Autodesk Inventor part; units mm, degrees
ref_plane "Flange Pattern Plane" through (19.05, 7.9375, -4.5466) normal (0, 1, 0) x (1, 0, 0)
ref_plane "YZ Plane" through (0, 0, 0) normal (1, 0, 0) x (0, 1, 0)
ref_plane "XZ Plane" through (0, 0, 0) normal (0, 1, 0) x (-1, 0, 0)
sketch "Sketch1" plane through (0, 0, 0) normal (0, 1, 0) x (-1, 0, 0)
  line L0 (-19.05, 0) -> (19.05, 0)
  line L1 (19.05, 0) -> (19.05, -25.4)
  line L2 (19.05, -25.4) -> (-19.05, -25.4)
  line L3 (-19.05, -25.4) -> (-19.05, 0)
  line L4 (19.05, 0) -> (-19.05, -25.4) construction
  point P0 (0, 0)
  point P1 (0, 0)
  dimension "d0" = 38.1
  dimension "d1" = 25.4
extrude "Plate1" add sketch "Sketch1" along normal blind 1.5875
sketch "Sketch2" plane through (17.4625, 0, -25.4) normal (1, 0, 0) x (0, 1, 0)
  line L0 (0, 25.4) -> (0, 0)
  line L1 (0, 0) -> (14.2875, 0)
  line L2 (14.2875, 0) -> (14.2875, 25.4)
  line L3 (14.2875, 25.4) -> (0, 25.4)
edge flange "Flanges" height 12.7 angle 90 thickness 1.5875 bend radius 0.7937 thickness toward (1, 0, 0) relief tear relief width 1.5875 relief depth 0.7937 corner gap 1.5875 corner form 0 edges at (19.05, 1.5875, -12.7) (-19.05, 1.5875, -12.7) wall of the first edge with corners at (17.4625, 0, 0) (17.4625, 0, -25.4) (17.4625, 14.2875, -25.4) (17.4625, 14.2875, 0)
bend "Bend1"
corner "Corner1"
sketch "Sketch3" plane through (19.05, 2.3813, -25.4) normal (1, 0, 0) x (0, 0, -1)
  line L0 (-20.8534, 7.8677) -> (-17.2466, 7.8677)
  line L1 (-16.7386, 7.3597) -> (-16.7386, 3.7529)
  line L2 (-17.2466, 3.2449) -> (-20.8534, 3.2449)
  line L3 (-21.3614, 3.7529) -> (-21.3614, 7.3597)
  arc A0 (-20.8534, 7.8677) -> (-21.3614, 7.3597) centre (-20.8534, 7.3597) ccw
  arc A1 (-16.7386, 7.3597) -> (-17.2466, 7.8677) centre (-17.2466, 7.3597) ccw
  arc A2 (-17.2466, 3.2449) -> (-16.7386, 3.7529) centre (-17.2466, 3.7529) ccw
  arc A3 (-21.3614, 3.7529) -> (-20.8534, 3.2449) centre (-20.8534, 3.7529) ccw
  line L4 (-25.4, 0) -> (-25.4, 11.9063) construction
  line L5 (-25.4, 11.9063) -> (0, 11.9062) construction
  line L6 (-20.8534, 7.3597) -> (-17.2466, 3.7529) construction
  point P0 (-25.4, -2.3812)
  point P1 (-16.7386, 3.2449)
  point P2 (-21.3614, 3.2449)
  point P3 (-19.05, 5.5563)
  dimension "d16" = 4.6228
  dimension "d17" = 0.508
  dimension "d20" = 6.35
  dimension "d21" = 6.35
extrude "Flange Stamp" cut sketch "Sketch3" against normal blind 1.5875
sketch "Sketch7" plane through (19.05, 2.3813, 0) normal (1, 0, 0) x (0, 0, -1)
  arc A0 (4.5466, 7.8677) -> (4.0386, 7.3597) centre (4.5466, 7.3597) ccw construction
  arc A1 (8.1534, 3.2449) -> (8.6614, 3.7529) centre (8.1534, 3.7529) ccw construction
  circle A2 centre (6.35, 5.5563) radius 2.1844
  line L0 (4.5466, 7.3597) -> (8.1534, 3.7529) construction
  point P0 (0, -2.3812)
  dimension "d46" = 4.3688
surface extrude "Flange Circle" sketch "Sketch7" against normal up to surface (1.5875 mm away) shown yes curves A2
ref_plane "Flange Pattern Plane" through (19.05, 7.9375, -4.5466) normal (0, 1, 0) x (1, 0, 0)
sketch "Flange Pattern Sketch" plane through (19.05, 7.9375, -4.5466) normal (0, 1, 0) x (1, 0, 0)
  line L0 (0, 3.6068) -> (0, 0) construction
  line L1 (-45.8186, -4.5466) -> (8.2118, -4.5466) construction
  line L2 (0, 0) -> (-1.5875, 0) construction
  point P0 (-19.05, -4.5466)
  point P1 (0, 1.8034)
  point P2 (0, 14.5034)
  dimension "d131" = 12.7
  dimension "d134" = 12.7
pattern_sketch "Flange Pattern" of "Flange Circle", "Flange Stamp" from (19.05, 7.9375, -6.35) copies at (19.05, 7.9375, -19.05)
sketch "Sketch8" plane through (0, 0, 0) normal (0, -1, 0) x (1, 0, 0)
  line L0 (16.6687, 0) -> (-16.6687, 0) construction
  line L1 (14.5034, -4.0386) -> (10.8966, -4.0386)
  line L2 (10.3886, -4.5466) -> (10.3886, -8.1534)
  line L3 (10.8966, -8.6614) -> (14.5034, -8.6614)
  line L4 (15.0114, -8.1534) -> (15.0114, -4.5466)
  arc A0 (15.0114, -4.5466) -> (14.5034, -4.0386) centre (14.5034, -4.5466) ccw
  arc A1 (14.5034, -8.6614) -> (15.0114, -8.1534) centre (14.5034, -8.1534) ccw
  arc A2 (10.3886, -8.1534) -> (10.8966, -8.6614) centre (10.8966, -8.1534) ccw
  arc A3 (10.8966, -4.0386) -> (10.3886, -4.5466) centre (10.8966, -4.5466) ccw
  line L5 (14.5034, -4.5466) -> (10.8966, -8.1534) construction
  line L6 (19.05, 0) -> (19.05, -25.4) construction
  point P0 (0, 0)
  point P1 (10.3886, -8.6614)
  point P2 (15.0114, -8.6614)
  point P3 (12.7, -6.35)
  dimension "d49" = 4.6228
  dimension "d50" = 0.508
  dimension "d51" = 6.35
  dimension "d52" = 6.35
extrude "Body Stamp" cut sketch "Sketch8" against normal blind 1.5875
sketch "Sketch9" plane through (0, 0, 0) normal (0, -1, 0) x (1, 0, 0)
  arc A0 (15.0114, -4.5466) -> (14.5034, -4.0386) centre (14.5034, -4.5466) ccw construction
  arc A1 (10.3886, -8.1534) -> (10.8966, -8.6614) centre (10.8966, -8.1534) ccw construction
  line L0 (14.5034, -4.5466) -> (10.8966, -8.1534) construction
  circle A2 centre (12.7, -6.35) radius 2.1844
  point P0 (0, 0)
  dimension "d55" = 4.3688
surface extrude "Body Circle" sketch "Sketch9" against normal up to surface (1.5875 mm away) shown yes curves A2
sketch "Body Pattern Sketch" plane through (0, 0, 0) normal (0, -1, 0) x (1, 0, 0)
  line L0 (16.6687, 0) -> (-16.6687, 0) construction
  line L1 (19.05, 0) -> (19.05, -25.4) construction
  circle A0 centre (12.7, -6.35) radius 2.1844 construction
  point P0 (0, 0)
  point P1 (12.7, -19.05)
  dimension "d62" = 12.7
  dimension "d65" = 12.7
  dimension "d139" = 12.7
pattern_sketch "Body Pattern" of "Body Stamp", "Body Circle" from (12.7, 0, -6.35) copies at (12.7, 0, -19.05)
sketch "Arc Length" plane through (17.4625, 2.3813, 0) normal (0, 0, 1) x (1, 0, 0)
  line L0 (0, 0) -> (1.5875, 0) construction
  arc A0 (-0.7937, -0.7938) -> (0, 0) centre (-0.7937, 0) ccw construction
  line L1 (-0.7938, -2.3813) -> (-0.7937, -0.7938) construction
  arc A1 (-0.7938, -2.3813) -> (1.5875, 0) centre (-0.7937, 0) ccw construction
  point P0 (-17.4625, -2.3812)
  dimension "d85" = 3.7405
  dimension "d92" = 1.2468
sketch "Sketch13" plane through (19.05, 14.2875, 0) normal (1, 0, 0) x (0, 0, -1)
  line L0 (0, 0) -> (25.4, 0) construction
  line L1 (62.4078, 0) -> (63.4238, -1.016)
  line L2 (63.4238, -1.016) -> (64.4398, 0)
  line L3 (62.4078, 0) -> (64.4398, 0)
  line L4 (25.4, -11.9062) -> (0, -11.9062) construction
  line L5 (63.4238, -10.8903) -> (61.161, -13.1531)
  line L6 (61.161, -13.1531) -> (63.4238, -15.4159)
  line L7 (63.4238, -15.4159) -> (65.6866, -13.1531)
  line L8 (65.6866, -13.1531) -> (63.4238, -10.8903)
  line L9 (63.4238, -10.8903) -> (63.4238, -15.4159) construction
  line L10 (63.4238, -1.016) -> (63.4238, -10.8903) construction
  line L11 (0, -11.9062) -> (25.4, -11.9062) construction
  point P0 (0, -14.2875)
  dimension "d86" = 4.5256
  dimension "d88" = 1.016
  dimension "d91" = 1.016
  dimension "d102" = 63.4238
feature "Notch" [suppressed]
mirror "Notch Mirror" [suppressed]
pattern_linear "Notch Pattern" [suppressed]
chamfer "End Chamfer" distance 1.016 angle 45 4 edges at (-18.2562, 14.2875, -25.4) (18.2563, 14.2875, -25.4) (-18.2562, 14.2875, 0) (18.2562, 14.2875, 0)
sketch "Sketch14" plane through (-19.05, 2.3813, 419.1) normal (1, 0, 0) x (0, 0, -1)
  line L0 (419.1, 11.9063) -> (444.5, 11.9063) construction
  line L1 (419.1, 0) -> (419.1, 11.9063) construction
  line L2 (419.1, -2.3813) -> (444.5, -2.3813) construction
  line L3 (419.1, 11.9063) -> (444.5, 11.9063)
  line L4 (444.5, 11.9063) -> (444.5, -2.3813)
  line L5 (444.5, -2.3813) -> (419.1, -2.3813)
  line L6 (419.1, -2.3813) -> (419.1, 11.9063)
  point P0 (419.1, -2.3812)
  point P1 (382.0521, -1.9844)
extrude "Half Cut" cut sketch "Sketch14" along normal blind 21.3614
equation "\"d1\" = 1.27 * Length"
equation "\"d18\" = Thickness"
equation "\"d53\" = Thickness"
equation "\"d89\" = Thickness"
equation "\"d2\" = Thickness"
equation "\"d3\" = BendReliefWidth"
equation "\"d4\" = BendReliefDepth"
equation "\"d5\" = MinimumRemnant"
equation "\"d6\" = TransitionRadius"
equation "\"d10\" = CornerReliefSize"
equation "\"d11\" = GapSize"
equation "\"d12\" = JacobiRadiusSize"
equation "\"BendRadius\" = Thickness"
equation "\"BendReliefWidth\" = Thickness"
equation "\"BendReliefDepth\" = 0.5 * Thickness"
equation "\"CornerReliefSize\" = 4 * Thickness"
equation "\"MinimumRemnant\" = 2 * Thickness"
equation "\"TransitionRadius\" = BendRadius"
equation "\"JacobiRadiusSize\" = BendRadius"
equation "\"GapSize\" = Thickness"
properties part number "Alu C 1x3x1x35"
The listing builds one solid part. Answer for the finished solid, in the listing's coordinates (mm). A direction names the side the tool comes from. Coordinates: 2 decimals unless noted, no trailing zeros. Write each loop counter-clockwise with the first axis right and the second up, starting at its lowest first coordinate (ties: lowest second). Pieces come first, ordered by that corner, then holes. Notation, with made-up numbers: M -9.5,39.25 L 39.5,39.25 A30 ccw 39.5,65.25 Z; hole C -25,69.5 d8. An arc over 180 degrees is marked long. Put each result on its own line as item: value. Start each with the question number.
1. A cutting plane is placed at D-D on x = 5.5. Write down the section's boundary in (y, z), then the cut area to 3 significant figures.
2. A cutting plane is placed at A-A on z = -19.5. Write down the section's boundary in (x, y).
3. A cutting plane is placed at C-C on y = 12.25. Write down the section's boundary in (x, z).
4. Which of the six approach directions +Z, -Z, +X, -X, +Y, -Y give full straight-line access (tool end or side, diameter ignored) to faces 1 (the flat face through (13, 1, -16.739)), 2 (the flat face through (18, 10.249, -19)), 3 (the flat face through (10, 1.588, -13)), 4 (the flat face through (18.27, 13.79, -24.88))?
5. Consider line 1 (Z direction, x = 18.25, y = 9.25); line 2 (X direction, y = 3.5, z = -19.25); line 3 (Y direction, x = 12.25, z = -8.75). Determine where each line is inside the solid, lowest interval first. Write a range as from..to.
6. For a pull along X with two mould halves and no side action, classify faces 5 (the flat face through (17.462, 8, -13)), 6 (the flat face through (15.011, 1, -19)), 7 (the flat face through (18, 8, -8.661)) as pulls with the +X half, pulls with the -X half, needs draft (parallel to the pull), parting line crosses it, or undercut.
7. A cutting plane is placed at B-B on z = -9.5. Write down the section's boundary in (x, y).
8. Flat-ended cylindrical pins translate along their axes: P1, Ø8, axis at y = 7.5, z = -22, coming from the -X side; P2, Ø0.8, axis at x = 18, z = -18.5, coming from the -Y side; P3, Ø0.8, axis at x = 18.5, y = 8, coming from the +Z side; P4, Ø1.7, axis at y = 1, z = -19, coming from the +X side. Find the tip coordinate at first contact, or state that the pin passes through.
Resolved:
1. outline: M 0,-25.4 L 1.59,-25.4 L 1.59,0 L 0,0 Z
1. area: 40.3 mm2
2. outline: M 2.31,0 L 10.39,0 L 10.39,1.59 L 2.31,1.59 Z; M 15.01,0 L 16.67,0 A2.38 ccw 19.05,2.38 L 19.05,5.63 L 17.46,5.63 L 17.46,2.38 A0.79 cw 16.67,1.59 L 15.01,1.59 Z; M 17.46,10.25 L 19.05,10.25 L 19.05,14.29 L 17.46,14.29 Z
3. outline: M 17.46,-25.4 L 19.05,-25.4 L 19.05,0 L 17.46,0 Z
4. face 1: +Y, -Y
4. face 2: +X, -X
4. face 3: +Z, -Z, -X, +Y
4. face 4: -Z, +X, -X, +Y
5. line 1: z = -25.4..-21.36, -16.74..-8.66, -4.04..0
5. line 2: x = 17.46..19.05
5. line 3: y = 0..1.59
6. face 5: pulls with the -X half
6. face 6: undercut
6. face 7: needs draft
7. outline: M 2.31,0 L 16.67,0 A2.38 ccw 19.05,2.38 L 19.05,14.29 L 17.46,14.29 L 17.46,2.38 A0.79 cw 16.67,1.59 L 2.31,1.59 Z
8. P1: stops at x = 17.46
8. P2: stops at y = 0.19
8. P3: stops at z = 0
8. P4: stops at x = 18.99
